```python
from build123d import *

# Parameters (mm, degrees)
DODANIE_WYCI_GNI_CIE1_DEPTH       = 2
WYCI_GNI_CIE_CIENKA_CIANKA1_DEPTH = 10
SZKIC3_R                          = 2.5
WYTNIJ_WYCI_GNI_CIE1_DEPTH        = 10


with BuildPart() as part:
    # Szkic1 → Dodanie-wyciągnięcie1 (new body)
    with BuildSketch(Plane(origin=(184.050171811, 0, -211.725502995), x_dir=(-0.75470958, 0, -0.656059029), z_dir=(0.656059029, 0, -0.75470958))):
        with BuildLine():
            Line((-985.697252828, -340.259541181), (-980.419174897, -315.823054253))
            Line((-980.419174897, -315.823054253), (-960.869985355, -320.045516598))
            Line((-960.869985355, -320.045516598), (-965.879501286, -343.238613058))
            add(Edge.make_bspline(
                [(-985.697252828, -340.259541181), (-980.093985624, -337.678026431), (-972.488962975, -338.490376385), (-965.879501286, -343.238613058)],
                knots=[0.113652907, 0.113652907, 0.113652907, 0.113652907, 0.285976573, 0.285976573, 0.285976573, 0.285976573], degree=3, weights=[0.648724237, 0.52341314, 0.477289897, 0.510354511]))
        make_face()
    extrude(amount=DODANIE_WYCI_GNI_CIE1_DEPTH)

    # Szkic2 → Wyciągnięcie-cienka ścianka1 (add)
    with BuildSketch(Plane(origin=(185.362289869, 0, -213.234922155), x_dir=(-0.75470958, 0, -0.656059029), z_dir=(0.656059029, 0, -0.75470958))):
        Polygon((-980.419174897, -315.823054253), (-960.869985355, -320.045516598), (-961.292231589, -322.000435553), (-980.841421131, -317.777973208), align=None)
    extrude(amount=WYCI_GNI_CIE_CIENKA_CIANKA1_DEPTH)

    # Szkic3 → Wytnij-wyciągnięcie1 (cut)
    with BuildSketch(Plane(origin=(82.487524873, -506.024310162, 71.705311407), x_dir=(-0.987224309, -0.157760609, 0.022355198), z_dir=(0.159336639, -0.977459477, 0.138509227))):
        with Locations((-849.886383223, -371.032714173)):
            Circle(SZKIC3_R)
    extrude(amount=-WYTNIJ_WYCI_GNI_CIE1_DEPTH, mode=Mode.SUBTRACT)


solid = part.part
```
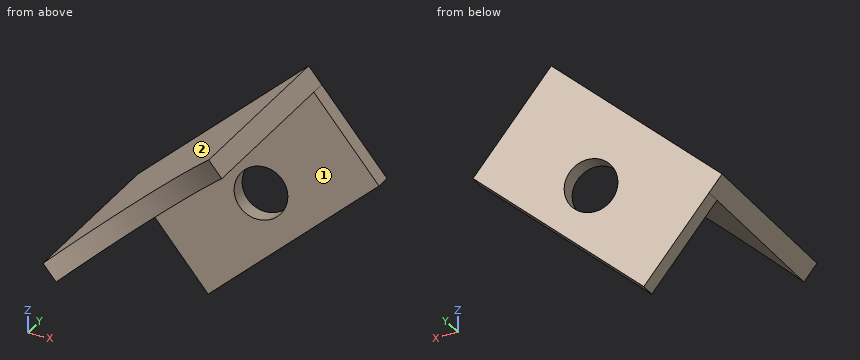
Geometry check sheet. Reference: the model listing, model coordinates, mm. Face numbers are marked on the shaded views. A direction names the side the tool comes from. Round coordinates to 2 decimals unless told otherwise and drop trailing zeros. Write each loop counter-clockwise with the first axis right and the second up, starting at its lowest first coordinate (ties: lowest second). Pieces come first, ordered by that corner, then holes. Notation, with made-up numbers: (-1.75, -1.5) -> (15.25, -1.5) arc R22 cw to (15.25, 6.5) -> close; hole circle Ø3 at (-1.5, 41). An arc over 180 degrees is marked (long way). Put each result on its own line as item: value.
1) Cross-section at B-B, the plane y = -326.25. Enter the section's corners in (x, z), plus the area to 3 significant figures.
Recorded:
outline: (910.24, 419.54) -> (911.55, 418.03) -> (926.99, 431.46) -> (925.68, 432.96) -> close
area: 40.9 mm2
2) Thickness scan on probe 1 along Y at (x, z) = (923.5, 428.25); probe 2 along Z at (x, y) = (911.75, -326); probe 3 along Z at (x, y) = (923.75, -336). Record the ranges inside material, lowest first. Write a range as from..to.
Recorded:
probe 1: y = -318.41..-316.36
probe 2: z = 418.2..420.85
probe 3: z = 428.64..431.29
3) Access from +Z, -Z, +X, -X, +Y, -Y to the whole of each face (thin tool, end or side, straight path). Record for the marked faces 1 and 2.
Recorded:
face 1: +X, -Y
face 2: +Z, -X, +Y, -Y
4) Depth check by flat-ended pin: P1, Ø3, axis at x = 929.5, z = 416, coming from the -Y side; P2, Ø8, axis at x = 924.5, y = -333.5, coming from the +Z side; P3, Ø1.5, axis at x = 928.5, y = -338, coming from the +Z side; P4, Ø2, axis at x = 929.5, z = 420.5, coming from the +Y side. Enter the tip coordinate at first touch or a pass-through.
Recorded:
P1: passes through
P2: stops at z = 434.39
P3: stops at z = 434.49
P4: stops at y = -316.26
5) Cross-section at A-A, the plane z = 416.5. Enter the section's corners in (x, y), plus the area to 3 significant figures.
Recorded:
outline: (911.11, -320.05) -> (911.67, -322) -> (925.03, -319.82) -> (925.03, -317.78) -> close
area: 27.9 mm2
